Read the model definition and answer for the solid it produces. Units are mm, in the model's axes. A direction names the side the tool comes from. Coordinates: 2 decimals unless noted, no trailing zeros. Order: outer loops, then holes, each group sorted by start corner. A loop starts at its lowest first (then second) coordinate and runs counter-clockwise, first axis right, second up.
```python
from build123d import *

# Parameters (mm, degrees)
BOSS_EXTRUDE1_DEPTH             = 14
CUT_EXTRUDE1_DEPTH              = 0.95
LPATTERN1_COUNT                 = 10
LPATTERN1_PITCH                 = 1.8
SKETCH3_R                       = 1.6
CUT_EXTRUDE2_DEPTH              = 21.976176963
SKETCH4_R                       = 5.4
BOSS_EXTRUDE2_DEPTH             = 7.65
BOSS_EXTRUDE3_REACH             = 32.332
SKETCH5_R                       = 4.5
SKETCH10_R                      = 2.5
CUT_EXTRUDE6_DEPTH              = 31.331501829
SKETCH9_R                       = 3.5
CUT_EXTRUDE5_DEPTH              = 17
M3X0_5_TAPPED_HOLE1_REACH       = 22.976
M3X0_5_TAPPED_HOLE1_BORE_R      = 1.25
M3X0_5_TAPPED_HOLE2_D           = 2.5
M3X0_5_TAPPED_HOLE2_DEPTH       = 4.15
M3X0_5_TAPPED_HOLE2_CSINK_D     = 3
M3X0_5_TAPPED_HOLE2_CSINK_ANGLE = 90


with BuildPart() as part:
    # Sketch1 → Boss-Extrude1 (new, symmetric)
    with BuildSketch(Plane(origin=(0, 0, 0), x_dir=(1, 0, 0), z_dir=(0, 1, 0))):
        with BuildLine():
            Line((-8, 6), (8, 6))
            ThreePointArc((8, 6), (10, 0), (8, -6))
            Line((8, -6), (-8, -6))
            ThreePointArc((-8, -6), (-10, 0), (-8, 6))
        make_face()
    extrude(amount=BOSS_EXTRUDE1_DEPTH, both=True)

    # Sketch2 → Cut-Extrude1 (cut)
    with BuildSketch(Plane(origin=(0, 7.3, 0), x_dir=(1, 0, 0), z_dir=(0, 1, 0))):
        with BuildLine():
            Line((8, 6), (-8, 6))
            ThreePointArc((-8, 6), (-10, 0), (-8, -6))
            Line((-8, -6), (8, -6))
            ThreePointArc((8, -6), (10, 0), (8, 6))
        make_face()
    cut_extrude1 = extrude(amount=-CUT_EXTRUDE1_DEPTH, mode=Mode.SUBTRACT)


with BuildPart() as cut_extrude1_piece_1:
    # of the separate pieces the step leaves, piece 1, a body of its own (cut_extrude1_pieces)
    add(part.part.solids().sort_by_distance((-8, -14, -6))[0])

    # LPattern1: Cut-Extrude1 ×10
    with Locations(*[(0, -i * LPATTERN1_PITCH, 0) for i in range(1, LPATTERN1_COUNT)]):
        add(cut_extrude1, mode=Mode.SUBTRACT)



with BuildPart() as cut_extrude1_piece_2:
    # of the separate pieces the step leaves, piece 2, a body of its own (cut_extrude1_pieces)
    add(part.part.solids().sort_by_distance((-8, 7.3, -6))[0])

    # Sketch3 → Cut-Extrude2 (cut, through all)
    with BuildSketch(Plane.XY.offset(6)):
        with Locations(Location((7, 10.5, 0), (0, 0, 308.682187453))):
            Circle(SKETCH3_R)
        with Locations(Location((-7, 10.5, 0), (0, 0, 128.682187453))):
            Circle(SKETCH3_R)
    extrude(amount=-CUT_EXTRUDE2_DEPTH, mode=Mode.SUBTRACT)


with BuildPart() as cut_extrude1_piece_1_1:
    add(cut_extrude1_piece_1.part)

    add(cut_extrude1_piece_2.part)  # Boss-Extrude2 merges Cut-Extrude1 piece 2
    # Sketch4 → Boss-Extrude2 (add)
    with BuildSketch(Plane(origin=(0, 14, 0), x_dir=(1, 0, 0), z_dir=(0, 1, 0))):
        with Locations(Location((0, 0, 0), (0, 0, 270))):
            Circle(SKETCH4_R)
    extrude(amount=-BOSS_EXTRUDE2_DEPTH)

    # Boss-Extrude3: up to this face of the body (flat: up to its plane)
    boss_extrude3_end = Plane(cut_extrude1_piece_1_1.part.faces().sort_by_distance((0, -9.85, 0))[0])
    # Sketch5 → Boss-Extrude3 (add, up to the picked face)
    with BuildSketch(Plane(origin=(0, 14, 0), x_dir=(1, 0, 0), z_dir=(0, 1, 0)), mode=Mode.PRIVATE) as boss_extrude3_sk1:
        with Locations(Location((0, 0, 0), (0, 0, 270))):
            Circle(SKETCH5_R)
    boss_extrude3_tool1 = split(extrude(boss_extrude3_sk1.sketch, amount=-BOSS_EXTRUDE3_REACH, mode=Mode.PRIVATE), bisect_by=boss_extrude3_end, keep=Keep.BOTH, mode=Mode.PRIVATE)
    add(boss_extrude3_tool1.solids().sort_by(Axis((0, 14, 0), (0, -1, 0)))[0])

    # Sketch7 → 1/8 NPT Tapped Hole1 (revolve, cut)
    with BuildSketch(Plane(origin=(0, 14, 0), x_dir=(0, 0, 1), z_dir=(1, 0, 0))):
        Polygon((0, 0), (0, 9.633468714), (4.2164, 7.1), (4.2164, 6.92), (4.953294211, 6.92), (5.143373, 0.571627), (5.715, 0), align=None)
    revolve(axis=Axis((0, 20.35, 0), (0, -1, 0)), mode=Mode.SUBTRACT)

    # Sketch10 → Cut-Extrude6 (cut, through all)
    with BuildSketch(Plane(origin=(0, 14, 0), x_dir=(1, 0, 0), z_dir=(0, 1, 0))):
        with Locations(Location((0, 0, 0), (0, 0, 270))):
            Circle(SKETCH10_R)
    extrude(amount=-CUT_EXTRUDE6_DEPTH, mode=Mode.SUBTRACT)

    # Sketch9 → Cut-Extrude5 (cut)
    with BuildSketch(Plane.XZ.offset(14)):
        with Locations(Location((0, 0, 0), (0, 0, 270))):
            Circle(SKETCH9_R)
    extrude(amount=-CUT_EXTRUDE5_DEPTH, mode=Mode.SUBTRACT)

    # M3x0.5 Tapped Hole1 bore → M3x0.5 Tapped Hole1 (cut, up to next)
    with BuildSketch(Plane(origin=(0, 0, 6), x_dir=(-1, 0, 0), z_dir=(0, 0, 1)), mode=Mode.PRIVATE) as m3x0_5_tapped_hole1_sk1:
        with Locations((0, 11.925)):
            Circle(M3X0_5_TAPPED_HOLE1_BORE_R)
    m3x0_5_tapped_hole1_tool1 = extrude(m3x0_5_tapped_hole1_sk1.sketch, amount=-M3X0_5_TAPPED_HOLE1_REACH, mode=Mode.PRIVATE) & cut_extrude1_piece_1_1.part
    add(m3x0_5_tapped_hole1_tool1.solids().sort_by_distance((0, -11.925, 6))[0], mode=Mode.SUBTRACT)

    # M3x0.5 Tapped Hole2
    with Locations(Plane(origin=(0, -14, 0), x_dir=(-1, 0, 0), z_dir=(0, -1, 0))):
        with Locations((6.85970884, 1.7), (-7, 1.7)):
            CounterSinkHole(M3X0_5_TAPPED_HOLE2_D / 2, M3X0_5_TAPPED_HOLE2_CSINK_D / 2, depth=M3X0_5_TAPPED_HOLE2_DEPTH, counter_sink_angle=M3X0_5_TAPPED_HOLE2_CSINK_ANGLE)


solid = cut_extrude1_piece_1_1.part
```
1) A cutting plane is placed at C-C, the plane y = -11.5. Determine the outline of the cut face in (x, z).
A:
outline: (-8, -6) - (8, -6) arc R10 ccw to (8, 6) - (1.18, 6) - (1.18, 3.3) arc R3.5 cw (long way) to (-1.18, 3.3) - (-1.18, 6) - (-8, 6) arc R10 ccw to start; hole circle Ø2.5 at (-6.86, -1.7); hole circle Ø2.5 at (7, -1.7)
2) A cutting plane is placed at A-A, the plane y = 10.5. Determine the outline of the cut face in (x, z).
A:
outline: (-8.6, -5.1) - (-8.6, 5.1) arc R10 ccw to start; (-5.4, -6) - (5.4, -6) - (5.4, 6) - (-5.4, 6) - close; (8.6, -5.1) arc R10 ccw to (8.6, 5.1) - close; hole circle Ø10.11 at (0, 0)
3) A cutting plane is placed at B-B, the plane x = 0. State how many separate pieces and enclosed holes the cut face has, and give its area (3 significant figures).
A:
separate pieces: 3
enclosed holes: 0
area: 90.9 mm2
4) Flat-ended cylindrical pins translate along their axes: pin 1 Ø3.5 at (x, z) = (-0.5, 0) entering from -Y; pin 2 Ø6 at (x, z) = (0, 0) entering from -Y. Find the tip coordinate at first contact, or state that the pin passes through.
A:
pin 1: passes through
pin 2: stops at y = 3
5) Straight lines are drawn through the part: line 1 (X direction, y = 3.8, z = 0); line 2 (X direction, y = 7, z = 0); line 3 (Z direction, x = 7, y = -11.15). For each, find the intervals that lie inside material, in ascending order.
A:
line 1: x = -10 to -2.5, 2.5 to 10
line 2: x = -5.4 to -4.22, 4.22 to 5.4
line 3: z = -6 to -2.95, -0.45 to 6
6) Determine the mould class of faces 3 (the cylindrical face through (1.352, -5.768, 4.292)), 4 (the cylindrical face through (-10, 2.3, 0.1)), 5 (the flat face through (0, 11, -6)), 6 (the cylindrical face through (-7.02, -11.77, -2.94)) for opening direction X: pulls with the +X half, pulls with the -X half, needs draft (parallel to the pull), parting line crosses it, or undercut.
A:
face 3: parting line crosses it
face 4: pulls with the -X half
face 5: needs draft
face 6: undercut
7) Which of the six approach directions +Z, -Z, +X, -X, +Y, -Y give full straight-line access (tool end or side, diameter ignored) to faces 1 (the cylindrical face through (1.352, 5.032, 4.292)), 2 (the cylindrical face through (-10, -3, 0))?
A:
face 1: none
face 2: -X, +Y, -Y
